```python
from build123d import *

# Parameters (mm, degrees)
ESQUISSE1_R        = 1
BOSS_EXTRU_1_DEPTH = 3


with BuildPart() as part:
    # Esquisse1 → Boss.-Extru.1 (new body)
    with BuildSketch(Plane(origin=(0, 0, 0), x_dir=(1, 0, 0), z_dir=(0, 1, 0))):
        with BuildLine():
            Line((-5, 46), (-5, 43))
            Line((-5, 43), (5, 43))
            Line((5, 43), (5, 46))
            Line((5, 46), (17, 46))
            Line((17, 46), (17, 3))
            ThreePointArc((17, 3), (16.121320344, 0.878679656), (14, 0))
            Line((14, 0), (-14, 0))
            ThreePointArc((-14, 0), (-16.121320344, 0.878679656), (-17, 3))
            Line((-17, 3), (-17, 46))
            Line((-17, 46), (-5, 46))
        make_face()
        with Locations(Location((0, 21, 0), (0, 0, 270))):
            Circle(ESQUISSE1_R, mode=Mode.SUBTRACT)
        with Locations(Location((-10, 21, 0), (0, 0, 270))):
            Circle(ESQUISSE1_R, mode=Mode.SUBTRACT)
        with Locations(Location((10, 21, 0), (0, 0, 270))):
            Circle(ESQUISSE1_R, mode=Mode.SUBTRACT)
    extrude(amount=BOSS_EXTRU_1_DEPTH)


solid = part.part
```
Work out the finished part from the listing and answer in its coordinate system (mm). A direction names the side the tool comes from. Round coordinates to 2 decimals unless told otherwise and drop trailing zeros. Write each loop counter-clockwise with the first axis right and the second up, starting at its lowest first coordinate (ties: lowest second). Pieces come first, ordered by that corner, then holes.
1) A cutting plane is placed at D-D on x = 10. Determine the outline of the cut face in (y, z), and give its area (3 significant figures).
2) Which of the six approach directions +Z, -Z, +X, -X, +Y, -Y give full straight-line access (tool end or side, diameter ignored) to faces 4 (the face through (-17, 1, -24)), 5 (the face through (5, 1, -44))?
3) A cutting plane is placed at B-B on x = 0. Determine the outline of the cut face in (y, z), and give its area (3 significant figures).
4) Consider probe 1 along X at (y, z) = (2.15, -21); probe 2 along Z at (x, y) = (0.5, 0.15); probe 3 along Z at (x, y) = (2.5, 1.9). Determine where each line is inside the solid, lowest interval first.
5) A cutting plane is placed at C-C on y = 2.2. Determine the outline of the cut face in (x, z), and give its area (3 significant figures).
6) A cutting plane is placed at A-A on z = -21. Determine the outline of the cut face in (x, y).
7) Determine the mould class of faces 1 (the face through (-5, 1, -45)), 2 (the face through (-11, 1, -46)), 3 (the face through (-16.1, 1.48, -0.86)) for opening direction X: pulls with the +X half, pulls with the -X half, needs draft (parallel to the pull), parting line crosses it, or undercut.
Entries:
1. outline: (0, -46) - (3, -46) - (3, -22) - (0, -22) - close; (0, -20) - (3, -20) - (3, 0) - (0, 0) - close
1. area: 132 mm2
2. face 4: +Z, -Z, -X, +Y, -Y
2. face 5: -Z, +Y, -Y
3. outline: (0, -43) - (3, -43) - (3, -22) - (0, -22) - close; (0, -20) - (3, -20) - (3, 0) - (0, 0) - close
3. area: 123 mm2
4. probe 1: x = -17 to -11, -9 to -1, 1 to 9, 11 to 17
4. probe 2: z = -43 to -21.87, -20.13 to 0
4. probe 3: z = -43 to 0
5. outline: (-17, -46) - (-5, -46) - (-5, -43) - (5, -43) - (5, -46) - (17, -46) - (17, -3) arc R3 ccw to (14, 0) - (-14, 0) arc R3 ccw to (-17, -3) - close; hole circle Ø2 at (-10, -21); hole circle Ø2 at (0, -21); hole circle Ø2 at (10, -21)
5. area: 1,520 mm2
6. outline: (-17, 0) - (-11, 0) - (-11, 3) - (-17, 3) - close; (-9, 0) - (-1, 0) - (-1, 3) - (-9, 3) - close; (1, 0) - (9, 0) - (9, 3) - (1, 3) - close; (11, 0) - (17, 0) - (17, 3) - (11, 3) - close
7. face 1: undercut
7. face 2: needs draft
7. face 3: pulls with the -X half
